from build123d import *

# Parameters (mm, degrees)
F1_DEPTH = 1
F2_DEPTH = 1


with BuildPart() as f1:
    # F0 (on Top) → F1 (new body)
    with BuildSketch(Plane.XY):
        with BuildLine():
            ThreePointArc((28.507673021, -4.2105263158), (28.0055681014, -2.6622878919), (26.5187842181, -2))
            Line((26.5187842181, -2), (-49.0589902927, -2))
            ThreePointArc((-49.0589902927, -2), (-50.5457741761, -2.6622878919), (-51.0478790956, -4.2105263158))
            ThreePointArc((-51.0478790956, -4.2105263158), (-11.2701030373, -40), (28.507673021, -4.2105263158))
        make_face()
        with BuildLine():
            ThreePointArc((26.5187842181, -2.7999999982), (27.4108545494, -3.1973727339), (27.7121175016, -4.1263157897))
            ThreePointArc((27.7121175016, -4.1263157897), (-11.2701030383, -39.2000000018), (-50.2523235764, -4.1263157876))
            ThreePointArc((-50.2523235764, -4.1263157876), (-49.9510606247, -3.1973727333), (-49.0589902947, -2.7999999982))
            Line((-49.0589902947, -2.7999999982), (26.5187842181, -2.7999999982))
        make_face(mode=Mode.SUBTRACT)
        with BuildLine():
            ThreePointArc((-50.2523235764, -4.1263157876), (-11.2701030383, -39.2000000018), (27.7121175016, -4.1263157897))
            ThreePointArc((27.7121175016, -4.1263157897), (27.4108545494, -3.1973727339), (26.5187842181, -2.7999999982))
            Line((26.5187842181, -2.7999999982), (-49.0589902947, -2.7999999982))
            ThreePointArc((-49.0589902947, -2.7999999982), (-49.9510606247, -3.1973727333), (-50.2523235764, -4.1263157876))
        make_face()
        with BuildLine():
            Line((-49.0589902947, -3.5999999382), (26.5187842181, -3.5999999382))
            ThreePointArc((26.5187842181, -3.5999999382), (26.8161410407, -3.732457537), (26.9165620401, -4.0421052697))
            ThreePointArc((26.9165620401, -4.0421052697), (-11.2701030383, -38.4000000618), (-49.456768115, -4.0421052677))
            ThreePointArc((-49.456768115, -4.0421052677), (-49.356347116, -3.7324575364), (-49.0589902947, -3.5999999382))
        make_face(mode=Mode.SUBTRACT)
        with BuildLine():
            ThreePointArc((26.9165620401, -4.0421052697), (26.8161410407, -3.732457537), (26.5187842181, -3.5999999382))
            Line((26.5187842181, -3.5999999382), (-49.0589902947, -3.5999999382))
            ThreePointArc((-49.0589902947, -3.5999999382), (-49.356347116, -3.7324575364), (-49.456768115, -4.0421052677))
            ThreePointArc((-49.456768115, -4.0421052677), (-11.2701030383, -38.4000000618), (26.9165620401, -4.0421052697))
        make_face()
    extrude(amount=F1_DEPTH)

    # F0 (on Top) → F2 (join)
    with BuildSketch(Plane.XY):
        with BuildLine():
            ThreePointArc((-50.2523235764, -4.1263157876), (-11.2701030383, -39.2000000018), (27.7121175016, -4.1263157897))
            ThreePointArc((27.7121175016, -4.1263157897), (27.4108545494, -3.1973727339), (26.5187842181, -2.7999999982))
            Line((26.5187842181, -2.7999999982), (-49.0589902947, -2.7999999982))
            ThreePointArc((-49.0589902947, -2.7999999982), (-49.9510606247, -3.1973727333), (-50.2523235764, -4.1263157876))
        make_face()
        with BuildLine():
            Line((-49.0589902947, -3.5999999382), (26.5187842181, -3.5999999382))
            ThreePointArc((26.5187842181, -3.5999999382), (26.8161410407, -3.732457537), (26.9165620401, -4.0421052697))
            ThreePointArc((26.9165620401, -4.0421052697), (-11.2701030383, -38.4000000618), (-49.456768115, -4.0421052677))
            ThreePointArc((-49.456768115, -4.0421052677), (-49.356347116, -3.7324575364), (-49.0589902947, -3.5999999382))
        make_face(mode=Mode.SUBTRACT)
    extrude(amount=-F2_DEPTH)


solid = f1.part
CAD build for the part. Positions are in the model's coordinates, mm. A direction names the side the tool comes from. Give positions to 0.01 mm unless a question says otherwise; leave off trailing zeros. Order: outer loops, then holes, each group sorted by start corner. A loop starts at its lowest first (then second) coordinate and runs counter-clockwise, first axis right, second up. Notation, with made-up numbers: (83.5, 24.25) - (103.5, 24.25) arc R19 cw to (103.5, 40.25) - close; hole circle Ø5 at (24.5, 75.25). An arc over 180 degrees is marked (long way). Answer in a Markdown table with one row per item.
1. Pull direction Y, two halves, no side cores. Call faces 1 (the flat face through (-12, -17, 1)), 2 (the cylindrical face through (-12.09, -39.99, 0.49)), 3 (the flat face through (-12, -17, 0)), 4 (the cylindrical face through (-10.48, -38.39, -0.49)): pulls with the +Y half, pulls with the -Y half, needs draft (parallel to the pull), parting line crosses it, or undercut.
Data:
| item | result |
|---|---|
| face 1 | needs draft |
| face 2 | pulls with the -Y half |
| face 3 | undercut |
| face 4 | undercut |
2. Saw through at C-C, the plane y = -31. Give the cut face in (x, z), plus the area to 3 significant figures.
Data:
| item | result |
|---|---|
| outline | (-36.55, 0) - (-35.26, 0) - (-35.26, -1) - (-33.93, -1) - (-33.93, 0) - (11.39, 0) - (11.39, -1) - (12.72, -1) - (12.72, 0) - (14.01, 0) - (14.01, 1) - (-36.55, 1) - close |
| area | 53.2 mm² |
3. Saw through at A-A, the plane z = -0.35. Give the cut face in (x, y), plus the area to 3 significant figures.
Data:
| item | result |
|---|---|
| outline | (-50.25, -4.13) arc R39.2 ccw to (27.71, -4.13) arc R1.2 ccw to (26.52, -2.8) - (-49.06, -2.8) arc R1.2 ccw to start; hole (-49.46, -4.04) arc R38.4 ccw to (26.92, -4.04) arc R0.4 ccw to (26.52, -3.6) - (-49.06, -3.6) arc R0.4 ccw to start |
| area | 154 mm² |
4. Saw through at B-B, the plane x = -12.5. Give the cut face in (y, z).
Data:
| item | result |
|---|---|
| outline | (-39.98, 0) - (-39.18, 0) - (-39.18, -1) - (-38.38, -1) - (-38.38, 0) - (-3.6, 0) - (-3.6, -1) - (-2.8, -1) - (-2.8, 0) - (-2, 0) - (-2, 1) - (-39.98, 1) - close |
5. Flat gauge pins, fed straight in: pin 1 (3 mm diameter, centred on x = -35.5, y = -8, fed in from -Z); pin 2 (1.1 mm diameter, centred on x = -17, z = -0.5, fed in from -Y); pin 3 (1.1 mm diameter, centred on x = 6, z = -0.5, fed in from +Y). Where does each tip first touch, or does it go through?
Data:
| item | result |
|---|---|
| pin 1 | stops at z = 0 |
| pin 2 | stops at y = -39.62 |
| pin 3 | stops at y = -2 |
6. Tool access for faces 5 (the cylindrical face through (-12.07, -39.19, -0.49)), 6 (the flat face through (-11, -3, -1)), 7 (the flat face through (-11.5, -2.6, 0)): list every direction of +Z, -Z, +X, -X, +Y, -Y with a clear straight run to the whole face (end or side of a thin tool).
Data:
| item | result |
|---|---|
| face 5 | -Z, -Y |
| face 6 | -Z, +X, -X, +Y, -Y |
| face 7 | -Z |
7. Probe probe 1 along Z at (x, y) = (-24.5, -24.5); probe 2 along X at (y, z) = (-10.5, -0.7); probe 3 along Y at (x, z) = (-28, -0.75). List the from-to ranges inside material, lowest first. Write a range as [from, to].
Data:
| item | result |
|---|---|
| probe 1 | z = [0, 1] |
| probe 2 | x = [-49.04, -48.21], [25.67, 26.5] |
| probe 3 | y = [-35.45, -34.56], [-3.6, -2.8] |
